Input: part model. Units: mm. Frame: model coordinates. Face numbers are marked on the shaded views. Give positions to 0.01 mm unless a question says otherwise; leave off trailing zeros. Order: outer loops, then holes, each group sorted by start corner. A loop starts at its lowest first (then second) coordinate and runs counter-clockwise, first axis right, second up. Notation, with made-up numbers: (-16.5, -18.5) - (3.5, -18.5) arc R37 ccw to (3.5, 17.5) - close; hole circle Ø2 at (-27, 20). An arc over 180 degrees is marked (long way). Answer in a Markdown table with one row per item. Add a question column.
from build123d import *

# Parameters (mm, degrees)
SKETCH_1_W      = 30
SKETCH_1_H      = 30
SKETCH_1_R      = 14.4
SKETCH_1_R_2    = 1.5
EXTRUDE_1_DEPTH = 10.3


with BuildPart() as part:
    # 草图1 → 凸台-拉伸1 (new body)
    with BuildSketch(Plane.XY):
        Rectangle(SKETCH_1_W, SKETCH_1_H)
        with Locations(Location((0, 0, 0), (0, 0, 180))):
            Circle(SKETCH_1_R, mode=Mode.SUBTRACT)
        with Locations(Location((-12, 12, 0), (0, 0, 180))):
            Circle(SKETCH_1_R_2, mode=Mode.SUBTRACT)
        with Locations(Location((12, 12, 0), (0, 0, 180))):
            Circle(SKETCH_1_R_2, mode=Mode.SUBTRACT)
        with Locations(Location((12, -12, 0), (0, 0, 180))):
            Circle(SKETCH_1_R_2, mode=Mode.SUBTRACT)
        with Locations(Location((-12, -12, 0), (0, 0, 180))):
            Circle(SKETCH_1_R_2, mode=Mode.SUBTRACT)
    extrude(amount=EXTRUDE_1_DEPTH)


solid = part.part
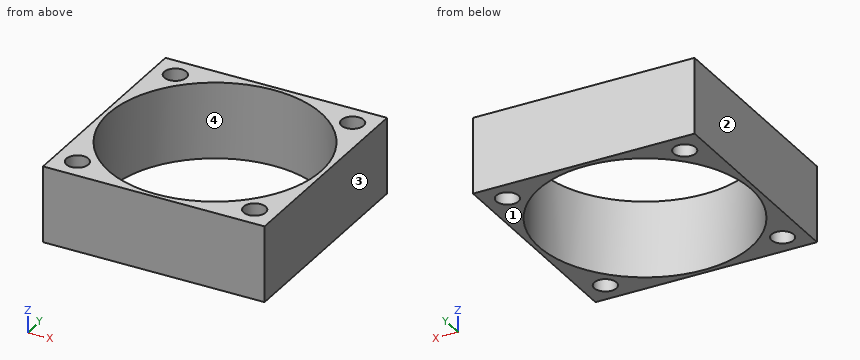
Q1. Section D-D, the plane x = -11. Return loops of the section in (y, z), then the cut area to 3 significant figures.
Q2. Pull-direction query (X, two-part tool) for the marked faces 1, 2, 3 and 4; classes: +X half, -X half, draft (parallel to the pull), parting line (faces both ways), or undercut.
Q3. Section A-A, the plane x = 0. Return loops of the section in (y, z).
Q4. Section C-C, the plane z = 9. Return loops of the section in (x, y), then the cut area to 3 significant figures.
Q5. Line query: probe 1 along Y at (x, z) = (12, 4.5); probe 2 along Y at (x, z) = (-12.25, 2.5). Output: solid intervals per line, ascending.
Q6. Contact query for a flat-ended pin moving along its axis: P1, Ø1.8, axis at x = 12, y = 12, coming from the +Z side. Output: stop coordinate, or through.
Computed:
| question | item | result |
|---|---|---|
| 1 | outline | (-15, 0) - (-13.12, 0) - (-13.12, 10.3) - (-15, 10.3) - close; (-10.88, 0) - (-9.29, 0) - (-9.29, 10.3) - (-10.88, 10.3) - close; (9.29, 0) - (10.88, 0) - (10.88, 10.3) - (9.29, 10.3) - close; (13.12, 0) - (15, 0) - (15, 10.3) - (13.12, 10.3) - close |
| 1 | area | 71.5 mm^2 |
| 2 | face 1 | draft |
| 2 | face 2 | -X half |
| 2 | face 3 | +X half |
| 2 | face 4 | undercut |
| 3 | outline | (-15, 0) - (-14.4, 0) - (-14.4, 10.3) - (-15, 10.3) - close; (14.4, 0) - (15, 0) - (15, 10.3) - (14.4, 10.3) - close |
| 4 | outline | (-15, -15) - (15, -15) - (15, 15) - (-15, 15) - close; hole circle Ø28.8 at (0, 0); hole circle Ø3 at (-12, -12); hole circle Ø3 at (-12, 12); hole circle Ø3 at (12, -12); hole circle Ø3 at (12, 12) |
| 4 | area | 220 mm^2 |
| 5 | probe 1 | y = -15 to -13.5, -10.5 to -7.96, 7.96 to 10.5, 13.5 to 15 |
| 5 | probe 2 | y = -15 to -13.48, -10.52 to -7.57, 7.57 to 10.52, 13.48 to 15 |
| 6 | P1 | passes through |
